from build123d import *

# Parameters (mm, degrees)
SKETCH1_W                  = 80
SKETCH1_H                  = 175
BOSS_EXTRUDE1_DEPTH        = 3.175
F_12_0MM_DOWEL_HOLE1_D     = 12
F_12_0MM_DOWEL_HOLE1_DEPTH = 3.175


with BuildPart() as part:
    # Sketch1 → Boss-Extrude1 (new body)
    with BuildSketch(Plane.XY):
        Rectangle(SKETCH1_W, SKETCH1_H)
    extrude(amount=BOSS_EXTRUDE1_DEPTH)

    # Ø12.0mm Dowel Hole1
    with Locations(Plane.XY.offset(3.175)):
        with Locations((0, 56.15)):
            Hole(F_12_0MM_DOWEL_HOLE1_D / 2, depth=F_12_0MM_DOWEL_HOLE1_DEPTH)


solid = part.part
Read the model definition and answer for the solid it produces. Units are mm, in the model's axes. Give positions to 0.01 mm unless a question says otherwise; leave off trailing zeros. Write each loop counter-clockwise with the first axis right and the second up, starting at its lowest first coordinate (ties: lowest second). Pieces come first, ordered by that corner, then holes. Notation, with made-up numbers: (62.25, 27.25) - (93.25, 27.25) arc R25 ccw to (93.25, 59.25) - close; hole circle Ø3 at (66, -18). An arc over 180 degrees is marked (long way). Return JSON: item names as keys, results as strings.
Q1. A cutting plane is placed at A-A, the plane x = 0. Determine the outline of the cut face in (y, z) (3 decimals).
Reply:
{"outline": "(-87.5, 0) - (50.15, 0) - (50.15, 3.175) - (-87.5, 3.175) - close; (62.15, 0) - (87.5, 0) - (87.5, 3.175) - (62.15, 3.175) - close"}
Q2. Consider line 1 along Y through (x, z) = (0, 2.3); line 2 along Y through (x, z) = (1.5, 0.3). Determine where each line is inside the solid, lowest interval first. Write a range as [from, to].
Reply:
{"line 1": "[-87.5, 50.15], [62.15, 87.5]", "line 2": "[-87.5, 50.34], [61.96, 87.5]"}
Q3. A cutting plane is placed at B-B, the plane y = 56.15. Determine the outline of the cut face in (x, z) (3 decimals), and give its area (3 significant figures).
Reply:
{"outline": "(-40, 0) - (-6, 0) - (-6, 3.175) - (-40, 3.175) - close; (6, 0) - (40, 0) - (40, 3.175) - (6, 3.175) - close", "area": "216 mm²"}
Q4. Given P1, Ø7, axis at x = 0, y = 56.15, coming from the +Z side, flat-ended and moving along its own axis, determine where the tip first touches the part or whether it passes through.
Reply:
{"P1": "through"}
Q5. For a pull along X with two mould halves and no side action, classify faces 1 (the face through (-1, -87.5, 2)), 2 (the face through (0.78, 62.1, 1.57)), 3 (the face through (-40, -1, 2)) as released by +X, released by -X, zero draft, split by the parting line, or undercut.
Reply:
{"face 1": "zero draft", "face 2": "undercut", "face 3": "released by -X"}
